Can you work these out from the model? Positions are in its coordinate system, mm. Give positions to 0.01 mm unless a question says otherwise; leave off trailing zeros. Loops run counter-clockwise (first coordinate to the right, second up) from the corner with the lowest first, then second, coordinate; pieces in that order, holes last.
from build123d import *

# Parameters (mm, degrees)
BOSS_EXTRUDE1_START = 12.7
SKETCH1_R           = 3.175
BOSS_EXTRUDE1_DEPTH = 2.032


with BuildPart() as part:
    # Sketch1 → Boss-Extrude1 (new body)
    with BuildSketch(Plane(origin=(0, 0, 0), x_dir=(0, 0, -1), z_dir=(1, 0, 0)).offset(BOSS_EXTRUDE1_START)):
        with BuildLine():
            Line((-10.015716817, -7.808675729), (-39.261787613, 29.703493203))
            ThreePointArc((-39.261787613, 29.703493203), (-40.308879957, 39.739856323), (-31.75, 45.085))
            Line((-31.75, 45.085), (10.015716817, 45.085))
            Line((10.015716817, 45.085), (10.015716817, 7.808675729))
            ThreePointArc((10.015716817, 7.808675729), (-7.808675729, 10.015716817), (-10.015716817, -7.808675729))
        make_face()
        with Locations((-31.75, 35.56)):
            Circle(SKETCH1_R, mode=Mode.SUBTRACT)
    extrude(amount=BOSS_EXTRUDE1_DEPTH)


solid = part.part
(1) Thinking about a two-plate mould opening in Z: for faces 1 (the cylindrical face through (13.7, 39.61, 40.37)), 2 (the flat face through (12.7, 25, 15)), 3 (the cylindrical face through (13.7, 32.46, 32.44)), which applies, pulls with the +Z half, pulls with the -Z half, needs draft (parallel to the pull), parting line crosses it, or undercut?
Returned:
face 1: pulls with the +Z half
face 2: needs draft
face 3: undercut
(2) Suppose I cut it at D-D on z = 0. List the corners of the cut face in (x, y) for me (3 decimals).
Returned:
outline: (12.7, 12.7) - (14.732, 12.7) - (14.732, 45.085) - (12.7, 45.085) - close
(3) Suppose I cut it at B-B on z = 32.5. List the corners of the cut face in (x, y) for me, plus the area to 3 significant figures.
Returned:
outline: (12.7, 21.03) - (14.73, 21.03) - (14.73, 32.47) - (12.7, 32.47) - close; (12.7, 38.65) - (14.73, 38.65) - (14.73, 45.06) - (12.7, 45.06) - close
area: 36.3 mm2
(4) Please list where these lines run through material, in increasing order: probe 1 along Y at (x, z) = (14.25, 31.75) (3 decimals); probe 2 along Z at (x, y) = (13.65, 35); probe 3 along Y at (x, z) = (13.35, 26) (3 decimals).
Returned:
probe 1: y = 20.069 to 32.385, 38.735 to 45.085
probe 2: z = -10.02 to 28.62, 34.88 to 41.26
probe 3: y = 12.693 to 45.085
(5) Will this pin go through, and if not, where does the flat tip stop? P1, Ø5, axis at y = 35.56, z = 31.75, coming from the +X side.
Returned:
P1: passes through
(6) Suppose I cut it at A-A on y = 35.56. List the corners of the cut face in (x, z) for me (3 decimals), plus the area to 3 significant figures.
Returned:
outline: (12.7, -10.016) - (14.732, -10.016) - (14.732, 28.575) - (12.7, 28.575) - close; (12.7, 34.925) - (14.732, 34.925) - (14.732, 41.275) - (12.7, 41.275) - close
area: 91.3 mm2
